Geometry: final body of the model. Coordinates: model frame, mm. Face numbers are marked on the shaded views. Give positions to 0.01 mm unless a question says otherwise; leave off trailing zeros. Loops run counter-clockwise (first coordinate to the right, second up) from the corner with the lowest first, then second, coordinate; pieces in that order, holes last.
1. Section B-B, the plane z = -15. Output: boundary loops of the cut face in (x, y), then the cut area to 3 significant figures.
2. Material intervals for line 1 along X through (y, z) = (2, -99); line 2 along Z through (x, y) = (256.55, 6.5); line 3 along Y through (x, z) = (120.5, -84), sorted ascending.
3. Section C-C, the plane x = 19. Output: boundary loops of the cut face in (y, z).
4. Draft query along X for the marked faces 1 and 2. Return one class per face: +X half, -X half, draft (parallel to the pull), parting line (faces both ways), or undercut.
5. Section A-A, the plane y = 11.75. Output: boundary loops of the cut face in (x, z), then the cut area to 3 significant figures.
6. First-contact query: P1, Ø2, axis at x = 99, z = -35, coming from the +Y side; P2, Ø4, axis at y = 6.5, z = -38, coming from the -X side. Flat tips, straight axial feed; report the tip coordinate or a pass-through.
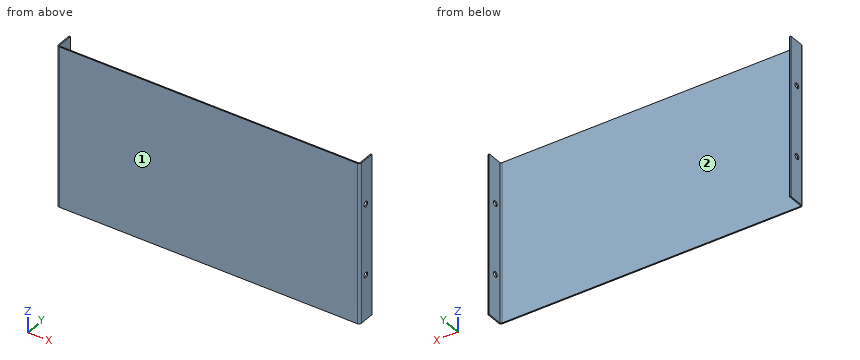
from build123d import *

# Parameters (mm, degrees)
SKETCH1_W                    = 256
SKETCH1_H                    = 136
BASE_FLANGE1_DEPTH           = 1
EDGE_FLANGE1_STRIP_W         = 6
EDGE_FLANGE1_STRIP_H         = 1
EDGE_FLANGE1_STRIP_CUT_DEPTH = 136
EDGE_FLANGE1_DEPTH           = 136
EDGE_FLANGE2_STRIP_W         = 6
EDGE_FLANGE2_STRIP_H         = 1
EDGE_FLANGE2_STRIP_CUT_DEPTH = 136
EDGE_FLANGE2_DEPTH           = 136
SKETCH12_R                   = 2.25
CUT_EXTRUDE1_DEPTH           = 278


# Sheet-metal steps are written as plain solids
with BuildPart() as part:
    # Sketch1 → Base-Flange1 (new body)
    with BuildSketch(Plane(origin=(0, 0, 0), x_dir=(1, 0, 0), z_dir=(0, 1, 0))):
        with Locations((128, 68)):
            Rectangle(SKETCH1_W, SKETCH1_H)
    extrude(amount=-BASE_FLANGE1_DEPTH)

    # Edge-Flange1 strip (across the edge) → Edge-Flange1 strip cut (cut)
    with BuildSketch(Plane.XY.offset(-136)):
        with Locations((-2, -0.5)):
            Rectangle(EDGE_FLANGE1_STRIP_W, EDGE_FLANGE1_STRIP_H)
    extrude(amount=EDGE_FLANGE1_STRIP_CUT_DEPTH, mode=Mode.SUBTRACT)

    # Edge-Flange1 section (across the edge) → Edge-Flange1 (add)
    with BuildSketch(Plane.XY.offset(-136)):
        with BuildLine():
            Line((-1, 1), (-1, 14))
            Line((-1, 14), (0, 14))
            Line((0, 14), (0, 1))
            ThreePointArc((0, 1), (0.292893219, 0.292893219), (1, 0))
            Line((1, 0), (1, -1))
            ThreePointArc((1, -1), (-0.414213562, -0.414213562), (-1, 1))
        make_face()
    extrude(amount=EDGE_FLANGE1_DEPTH)

    # Edge-Flange2 strip (across the edge) → Edge-Flange2 strip cut (cut)
    with BuildSketch(Plane(origin=(256, 0, 0), x_dir=(-1, 0, 0), z_dir=(0, 0, -1))):
        with Locations((-2, -0.5)):
            Rectangle(EDGE_FLANGE2_STRIP_W, EDGE_FLANGE2_STRIP_H)
    extrude(amount=EDGE_FLANGE2_STRIP_CUT_DEPTH, mode=Mode.SUBTRACT)

    # Edge-Flange2 section (across the edge) → Edge-Flange2 (add)
    with BuildSketch(Plane(origin=(256, 0, 0), x_dir=(-1, 0, 0), z_dir=(0, 0, -1))):
        with BuildLine():
            Line((-1, 1), (-1, 14))
            Line((-1, 14), (0, 14))
            Line((0, 14), (0, 1))
            ThreePointArc((0, 1), (0.292893219, 0.292893219), (1, 0))
            Line((1, 0), (1, -1))
            ThreePointArc((1, -1), (-0.414213562, -0.414213562), (-1, 1))
        make_face()
    extrude(amount=EDGE_FLANGE2_DEPTH)

    # Sketch12 → Cut-Extrude1 (cut)
    with BuildSketch(Plane(origin=(-2, -333.400026456, -193.062536038), x_dir=(0, 1, 0), z_dir=(-1, 0, 0))):
        with Locations(Location((339.900026456, -95.062536038, 0), (0, 0, 180))):
            Circle(SKETCH12_R)
        with Locations(Location((339.900026456, -155.062536038, 0), (0, 0, 180))):
            Circle(SKETCH12_R)
    extrude(amount=-CUT_EXTRUDE1_DEPTH, mode=Mode.SUBTRACT)


solid = part.part
Answers below:
1. outline: (-1, 1) arc R2 ccw to (1, -1) - (255, -1) arc R2 ccw to (257, 1) - (257, 14) - (256, 14) - (256, 1) arc R1 cw to (255, 0) - (1, 0) arc R1 cw to (0, 1) - (0, 14) - (-1, 14) - close
1. area: 285 mm2
2. line 1: x = -1 to 0, 256 to 257
2. line 2: z = -136 to -100.25, -95.75 to -40.25, -35.75 to 0
2. line 3: y = -1 to 0
3. outline: (-1, -136) - (0, -136) - (0, 0) - (-1, 0) - close
4. face 1: draft
4. face 2: undercut
5. outline: (-1, -136) - (0, -136) - (0, 0) - (-1, 0) - close; (256, -136) - (257, -136) - (257, 0) - (256, 0) - close
5. area: 272 mm2
6. P1: stops at y = 0
6. P2: passes through
